Design review of the part built by this model. Coordinates are the model's own, in mm. Face numbers are marked on the shaded views. A direction names the side the tool comes from. Give positions to 0.01 mm unless a question says otherwise; leave off trailing zeros. Write each loop counter-clockwise with the first axis right and the second up, starting at its lowest first coordinate (ties: lowest second). Pieces come first, ordered by that corner, then holes.
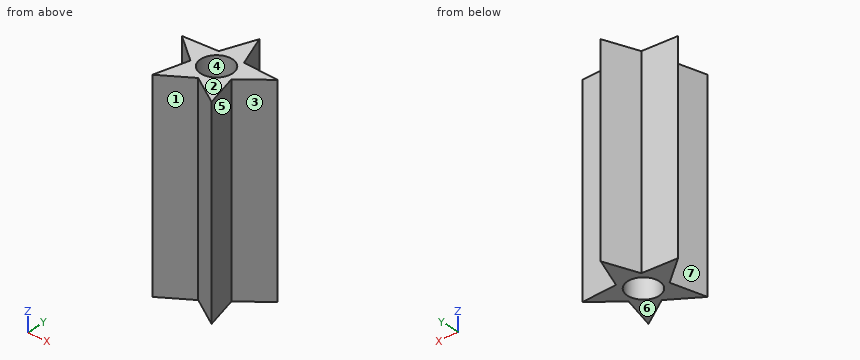
```python
from build123d import *

# Parameters (mm, degrees)
BOSS_EXTRUDE1_DEPTH = 70
SKETCH2_R           = 5.5
CUT_EXTRUDE1_DEPTH  = 75.049008955


with BuildPart() as part:
    # Sketch1 → Boss-Extrude1 (new body)
    with BuildSketch(Plane.XY):
        Polygon((0, 17.5), (-4.408389392, 6.067627458), (-16.643489035, 5.407797402), (-7.132923872, -2.317627458), (-10.286241915, -14.157797402), (0, -7.5), (10.286241915, -14.157797402), (7.132923872, -2.317627458), (16.643489035, 5.407797402), (4.408389392, 6.067627458), align=None)
    extrude(amount=BOSS_EXTRUDE1_DEPTH)

    # Sketch2 → Cut-Extrude1 (cut, through all)
    with BuildSketch(Plane.XY.offset(70)):
        Circle(SKETCH2_R)
    extrude(amount=-CUT_EXTRUDE1_DEPTH, mode=Mode.SUBTRACT)


solid = part.part
```
(1) To check wall thickness, follow L1, parallel to Y at x = -5, z = 46; L2, parallel to X at y = -10.5, z = 13.5; L3, parallel to X at y = -2.5, z = 30.5. State the ranges of each line that lie inside material, in increasing order.
Resolved:
L1: y = -10.74 to -2.29, 2.29 to 6.04
L2: x = -9.31 to -4.63, 4.63 to 9.31
L3: x = -7.18 to -4.9, 4.9 to 7.18
(2) Mouldability with a two-part tool opening along X and no side actions: class the marked faces 1, 2, 3 and 4 as pulls with the +X half, pulls with the -X half, needs draft (parallel to the pull), parting line crosses it, or undercut.
Resolved:
face 1: undercut
face 2: needs draft
face 3: pulls with the +X half
face 4: undercut
(3) Tool access review of the marked faces 5, 6 and 7: name each direction out of +Z, -Z, +X, -X, +Y, -Y from which nothing blocks a thin tool from reaching the whole face with its end or side.
Resolved:
face 5: +Z, -Z, +X
face 6: -Z, +X, -X, +Y, -Y
face 7: +Z, -Z, -X
(4) Consider section B-B, the plane y = 2. Give the boundary of the cut face in (x, z).
Resolved:
outline: (-12.45, 0) - (-5.12, 0) - (-5.12, 70) - (-12.45, 70) - close; (5.12, 0) - (12.45, 0) - (12.45, 70) - (5.12, 70) - close
(5) Consider section D-D, the plane x = 14.5. Give the boundary of the cut face in (y, z).
Resolved:
outline: (3.67, 0) - (5.52, 0) - (5.52, 70) - (3.67, 70) - close
(6) Consider section A-A, the plane z = 22. Give the boundary of the cut face in (x, y).
Resolved:
outline: (-16.64, 5.41) - (-7.13, -2.32) - (-10.29, -14.16) - (0, -7.5) - (10.29, -14.16) - (7.13, -2.32) - (16.64, 5.41) - (4.41, 6.07) - (0, 17.5) - (-4.41, 6.07) - close; hole circle Ø11 at (0, 0)
(7) Consider section C-C, the plane x = -2. Give the boundary of the cut face in (y, z).
Resolved:
outline: (-8.79, 0) - (-5.12, 0) - (-5.12, 70) - (-8.79, 70) - close; (5.12, 0) - (12.31, 0) - (12.31, 70) - (5.12, 70) - close
(8) Clearance check with flat-ended pins moving along their axes: P1, Ø1.5, axis at y = -7, z = 25, coming from the -X side; P2, Ø8, axis at y = 13.5, z = 22, coming from the -X side; P3, Ø2, axis at y = -3.5, z = 58.5, coming from the -X side. State where each tip first meets the part, or that it passes through.
Resolved:
P1: stops at x = -8.58
P2: stops at x = -3.08
P3: stops at x = -7.71
